The drawing under review shows one solid part. Ordinate dimensions are in mm from its lowest x, y, z. Round coordinates to 2 decimals unless told otherwise and drop trailing zeros. Write each loop counter-clockwise with the first axis right and the second up, starting at its lowest first coordinate (ties: lowest second). Pieces come first, ordered by that corner, then holes. Notation, with made-up numbers: M 45.25,4 L 89.25,4 A22 ccw 89.25,35 Z; hole C 26.5,-32 d4. An arc over 180 degrees is marked long. Write item = value, one per line. Start each with the question number.
Item 1: To check wall thickness, follow line 1 along X through (y, z) = (40.5, 22); line 2 along Z through (x, y) = (4.5, 6.5); line 3 along X through (y, z) = (6, 37.5). State the ranges of each line that lie inside material, in increasing order.
Item 2: Take a section at A-A, the plane x = 5. Give the boundary of the cut face in (y, z).
Item 3: Take a section at C-C, the plane y = 6. Give the boundary of the cut face in (x, z), plus the area to 3 significant figures.
Item 4: For pin 1 Ø2 at (x, z) = (2.5, 31) entering from -Y; pin 2 Ø6 at (x, z) = (21, 15) entering from -Y; pin 3 Ø2 at (y, z) = (2.5, 29) entering from -X; pin 4 Ø2 at (y, z) = (41.5, 36) entering from +X, all flat-tipped, find the tip position at first contact; note any pin that passes through.
Item 5: Take a section at B-B, the plane z = 33.5. Give the boundary of the cut face in (x, y).
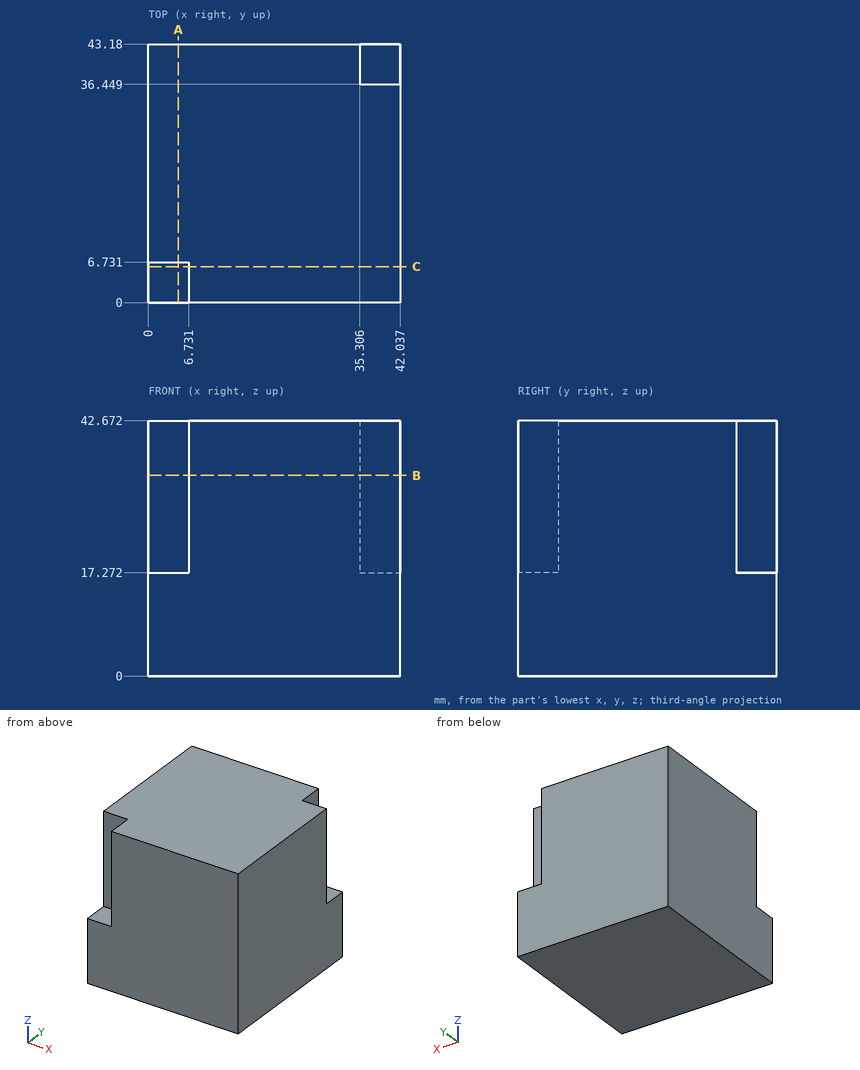
Response values:
q1.line_1 = 0 to 35.31
q1.line_2 = 0 to 17.27
q1.line_3 = 6.73 to 42.04
q2.outline = M 0,0 L 43.18,0 L 43.18,42.67 L 6.73,42.67 L 6.73,17.27 L 0,17.27 Z
q3.outline = M 0,0 L 42.04,0 L 42.04,42.67 L 6.73,42.67 L 6.73,17.27 L 0,17.27 Z
q3.area = 1,620 mm2
q4.pin_1 = 6.73
q4.pin_2 = 0
q4.pin_3 = 6.73
q4.pin_4 = 35.31
q5.outline = M 0,6.73 L 6.73,6.73 L 6.73,0 L 42.04,0 L 42.04,36.45 L 35.31,36.45 L 35.31,43.18 L 0,43.18 Z
